Can you work these out from the model? Positions are in its coordinate system, mm. Face numbers are marked on the shaded views. Give positions to 0.01 mm unless a question says otherwise; leave off trailing zeros. Order: outer loops, then holes, each group sorted by start corner. A loop starts at its lowest first (then second) coordinate and runs counter-clockwise, first axis right, second up. Notation, with made-up numbers: (69.5, -14.75) - (125.5, -14.75) arc R27 ccw to (125.5, 24.25) - close; hole circle Ø1 at (1.25, -27.75). An arc over 180 degrees is marked (long way). Answer as a JSON object with one key per item and string values.
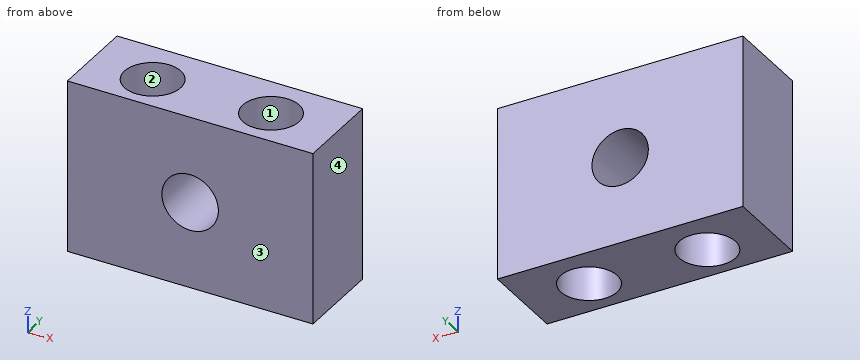
```python
from build123d import *

# Parameters (mm, degrees)
F0_W     = 71.80953
F0_H     = 50.532632
F1_DEPTH = 25.4
F3_D     = 16.51
F5_D     = 16.51


with BuildPart() as f1:
    # F0 (on Front) → F1 (new body)
    with BuildSketch(Plane.XZ):
        Rectangle(F0_W, F0_H)
    extrude(amount=F1_DEPTH)

    # F3 (through all)
    with Locations(Plane.XZ.offset(25.4)):
        with Locations((0, 0)):
            Hole(F3_D / 2)

    # F5 (through all)
    with Locations(Plane.XY.offset(25.266316)):
        with Locations((-17.509114, -13.962964), (16.844211, -13.519696)):
            Hole(F5_D / 2)


solid = f1.part
```
Q1. We'd pull the mould along Y, two halves only. Please class the marked faces 1, 2, 3 and 4: released by +Y, released by -Y, zero draft, split by the parting line, or undercut.
Recorded:
{"face 1": "undercut", "face 2": "undercut", "face 3": "released by -Y", "face 4": "zero draft"}
Q2. I need wall thicknesses on L1, parallel to Y at x = 16.5, z = -11; L2, parallel to X at y = -10.25, z = -14; L3, parallel to Z at x = 0, y = -16.5 (3 decimals). Which ranges of each line are inside material? Lowest first, please.
Recorded:
{"L1": "y = -25.4 to -21.77, -5.27 to 0", "L2": "x = -35.9 to -24.88, -10.14 to 9.26, 24.42 to 35.9", "L3": "z = -25.266 to -8.255, 8.255 to 25.266"}
Q3. If we section it at B-B, the plane z = 0: Please give me the cut outline in (x, y) (3 decimals), then the cut area to 3 significant figures.
Recorded:
{"outline": "(-35.905, -25.4) - (-8.255, -25.4) - (-8.255, 0) - (-35.905, 0) - close; (8.255, -25.4) - (35.905, -25.4) - (35.905, 0) - (8.255, 0) - close; hole circle Ø16.51 at (-17.509, -13.963); hole circle Ø16.51 at (16.844, -13.52)", "area": "976 mm^2"}
Q4. If we section it at D-D, the plane y = -23.5: Please give me the cut outline in (x, z) (3 decimals).
Recorded:
{"outline": "(-35.905, -25.266) - (35.905, -25.266) - (35.905, 25.266) - (-35.905, 25.266) - close; hole circle Ø16.51 at (0, 0)"}
Q5. If we section it at C-C, the plane x = 0: Please give me the cut outline in (y, z) (3 decimals).
Recorded:
{"outline": "(-25.4, -25.266) - (0, -25.266) - (0, -8.255) - (-25.4, -8.255) - close; (-25.4, 8.255) - (0, 8.255) - (0, 25.266) - (-25.4, 25.266) - close"}
Q6. If we section it at A-A, the plane y = -17.25: Please give me the cut outline in (x, z) (3 decimals), then the cut area to 3 significant figures.
Recorded:
{"outline": "(-35.905, -25.266) - (-25.081, -25.266) - (-25.081, 25.266) - (-35.905, 25.266) - close; (-9.937, -25.266) - (9.48, -25.266) - (9.48, 25.266) - (-9.937, 25.266) - close; (24.208, -25.266) - (35.905, -25.266) - (35.905, 25.266) - (24.208, 25.266) - close; hole circle Ø16.51 at (0, 0)", "area": "1,910 mm^2"}
